Source: CAD feature listing. Evaluate the final solid. Frame: model axes, mm. Face numbers are marked on the shaded views. A direction names the side the tool comes from. Give positions to 0.01 mm unless a question says otherwise; leave off trailing zeros. Order: outer loops, then holes, each group sorted by start corner. A loop starts at its lowest first (then second) coordinate and runs counter-clockwise, first axis right, second up. Notation, with made-up numbers: M -9,33 L 3,33 A16 cw 3,39 Z; hole C 77,11.25 d7. An arc over 180 degrees is marked long. Answer as a JSON object with one key per item and string values. Group by question number.
1. Section query A-A (z = -20.5). Output: boundary loops of the cut face in (x, y), plus the area to 3 significant figures.
2. Section query B-B (x = 8.5). Output: boundary loops of the cut face in (y, z).
3. Section query C-C (y = 5.25). Output: boundary loops of the cut face in (x, z).
4. Material intervals for L1, parallel to Z at x = -34, y = 22.5; L2, parallel to X at y = 6.25, z = -21.5; L3, parallel to Y at x = -19, z = -27, sorted ascending. Write a range as [from, to].
5. Pin query (flat end, axial travel): P1, Ø13, axis at y = 14, z = 25.5, coming from the -X side; P2, Ø5, axis at x = -24, y = 10, coming from the -Z side; P3, Ø8, axis at y = 18.5, z = -20, coming from the +X side. Return the tip coordinate at first contact, or that it passes through.
6. Set-up query: the marked faces 1, 2, 3, 4 and 5. Return all of +Z, -Z, +X, -X, +Y, -Y with unobstructed straight access to the full face (end or side cutting, diameter ignored); none if empty.
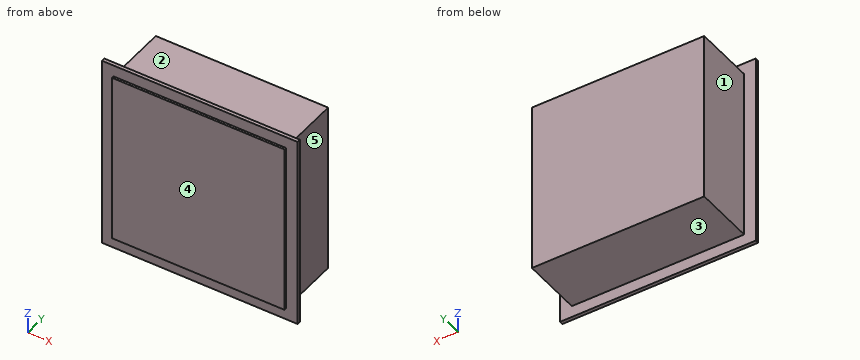
from build123d import *

# Parameters (mm, degrees)
SKETCH_1_W      = 84
SKETCH_1_H      = 84
EXTRUDE_1_DEPTH = 1.5
SKETCH_2_W      = 74
SKETCH_2_H      = 74
EXTRUDE_2_DEPTH = 26
SKETCH_3_W      = 74
SKETCH_3_H      = 74
EXTRUDE_3_DEPTH = 1


with BuildPart() as part:
    # 草图1 → 凸台-拉伸1 (new body)
    with BuildSketch(Plane(origin=(0, 0, 0), x_dir=(1, 0, 0), z_dir=(0, 1, 0))):
        with Locations((1.82278481, -10.17721519)):
            Rectangle(SKETCH_1_W, SKETCH_1_H)
    extrude(amount=EXTRUDE_1_DEPTH)

    # 草图2 → 凸台-拉伸2 (add)
    with BuildSketch(Plane(origin=(0, 1.5, 0), x_dir=(1, 0, 0), z_dir=(0, 1, 0))):
        with Locations((1.82278481, -10.17721519)):
            Rectangle(SKETCH_2_W, SKETCH_2_H)
    extrude(amount=EXTRUDE_2_DEPTH)

    # 草图3 → 凸台-拉伸3 (add)
    with BuildSketch(Plane.XZ):
        with Locations((1.82278481, 10.17721519)):
            Rectangle(SKETCH_3_W, SKETCH_3_H)
    extrude(amount=EXTRUDE_3_DEPTH)


solid = part.part
Answer sheet:
{
 "1": {"outline": "M -40.18,0 L -35.18,0 L -35.18,-1 L 38.82,-1 L 38.82,0 L 43.82,0 L 43.82,1.5 L 38.82,1.5 L 38.82,27.5 L -35.18,27.5 L -35.18,1.5 L -40.18,1.5 Z", "area": "2,120 mm^2"},
 "2": {"outline": "M -1,-26.82 L 0,-26.82 L 0,-31.82 L 1.5,-31.82 L 1.5,-26.82 L 27.5,-26.82 L 27.5,47.18 L 1.5,47.18 L 1.5,52.18 L 0,52.18 L 0,47.18 L -1,47.18 Z"},
 "3": {"outline": "M -35.18,-26.82 L 38.82,-26.82 L 38.82,47.18 L -35.18,47.18 Z"},
 "4": {"L1": "[-26.82, 47.18]", "L2": "[-35.18, 38.82]", "L3": "[0, 1.5]"},
 "5": {"P1": "x = -35.18", "P2": "z = -26.82", "P3": "x = 38.82"},
 "6": {"face 1": "+Z, -Z, -X, +Y", "face 2": "+Z, +X, -X, +Y", "face 3": "-Z, +X, -X, +Y", "face 4": "+Z, -Z, +X, -X, -Y", "face 5": "+Z, -Z, +X, +Y"}
}
